from build123d import *

# Parameters (mm, degrees)
F0_W     = 70
F0_H     = 65
F1_DEPTH = 1.5
F2_W     = 5
F2_H     = 51
F3_DEPTH = 11
F4_W     = 70
F4_H     = 65
F5_DEPTH = 1.5
F6_R     = 1.5
F7_DEPTH = 25
F8_R     = 1
F9_DEPTH = 15.2


with BuildPart() as f1:
    # F0 (on Front) → F1 (new body)
    with BuildSketch(Plane.XZ):
        with Locations((35, 32.5)):
            Rectangle(F0_W, F0_H)
    extrude(amount=-F1_DEPTH)

    # F2 (on face) → F3 (join)
    with BuildSketch(Plane(origin=(0, 1.5, 0), x_dir=(-1, 0, 0), z_dir=(0, 1, 0))):
        with Locations((-67.5, 32.5)):
            Rectangle(F2_W, F2_H)
        with Locations((-2.5, 32.5)):
            Rectangle(F2_W, F2_H)
    extrude(amount=F3_DEPTH)

    # F4 (on face) → F5 (join)
    with BuildSketch(Plane(origin=(0, 12.5, 0), x_dir=(-1, 0, 0), z_dir=(0, 1, 0))):
        with Locations((-35, 32.5)):
            Rectangle(F4_W, F4_H)
    extrude(amount=F5_DEPTH)

    # F6 (on Front) → F7 (cut)
    with BuildSketch(Plane.XZ):
        with Locations((3, 62)):
            Circle(F6_R)
        with Locations((67, 62)):
            Circle(F6_R)
        with Locations((3, 3)):
            Circle(F6_R)
        with Locations((67, 3)):
            Circle(F6_R)
    extrude(amount=-F7_DEPTH, mode=Mode.SUBTRACT)

    # F8 (on face) → F9 (join)
    with BuildSketch(Plane.XZ):
        Polygon((5.75, 60.412287), (5.75, 63.587713), (3, 65.175426), (0.25, 63.587713), (0.25, 60.412287), (3, 58.824574), align=None)
        with Locations((3, 62)):
            Circle(F8_R, mode=Mode.SUBTRACT)
        Polygon((5.75, 1.412287), (5.75, 4.587713), (3, 6.175426), (0.25, 4.587713), (0.25, 1.412287), (3, -0.175426), align=None)
        with Locations((3, 3)):
            Circle(F8_R, mode=Mode.SUBTRACT)
        Polygon((67, 58.824574), (69.75, 60.412287), (69.75, 63.587713), (67, 65.175426), (64.25, 63.587713), (64.25, 60.412287), align=None)
        with Locations((67, 62)):
            Circle(F8_R, mode=Mode.SUBTRACT)
        Polygon((67, -0.175426), (69.75, 1.412287), (69.75, 4.587713), (67, 6.175426), (64.25, 4.587713), (64.25, 1.412287), align=None)
        with Locations((67, 3)):
            Circle(F8_R, mode=Mode.SUBTRACT)
    extrude(amount=F9_DEPTH)


solid = f1.part
Source: CAD feature listing. Evaluate the final solid. Frame: model axes, mm. A direction names the side the tool comes from. Round coordinates to 2 decimals unless told otherwise and drop trailing zeros. Loops run counter-clockwise (first coordinate to the right, second up) from the corner with the lowest first, then second, coordinate; pieces in that order, holes last.
Q1. Section B-B, the plane x = 58. Return loops of the section in (y, z), plus the area to 3 significant figures.
Q2. Section C-C, the plane z = 29.5. Return loops of the section in (x, y), plus the area to 3 significant figures.
Q3. Section D-D, the plane y = 4. Return loops of the section in (x, z), plus the area to 3 significant figures.
Q4. Section A-A, the plane y = -9.5. Return loops of the section in (x, z), plus the area to 3 significant figures.
Q5. First-contact query: P1, Ø12, axis at x = 14.5, z = 15.5, coming from the -Y side; P2, Ø3.5, axis at y = -11.5, z = 61.5, coming from the +X side; P3, Ø1, axis at y = -11.5, z = 61, coming from the -X side; P4, Ø4, axis at x = 3, z = 62, coming from the +Y side. Flat tips, straight axial feed; report the tip coordinate or a pass-through.
Q6. Access query for faces 5 (the face through (4.394, -7.494, 5.37)), 6 (the face through (4.36, -7.49, 0.61)), 7 (the face through (2.805, 13.24, 63.487)). Directions: +Z, -Z, +X, -X, +Y, -Y. A direction counts if a zero-diameter tool reaches every point of the face in a straight line with its end or side. Return the directions, or none.
Q7. Ray query, line 1 (Z direction, x = 3, y = -3); line 2 (Z direction, x = 3, y = 0.45); line 3 (Y direction, x = 32, z = 44). Return the intervals inside material, ascending.
Q8. Mould query, pull axis X, two halves, no side actions, for faces 1 (the face through (1.606, -7.494, 0.63)), 2 (the face through (68.394, -7.494, 64.37)), 3 (the face through (65, 7, 32)), 4 (the face through (3, 7, 58)). Classes: pulls with the +X half, pulls with the -X half, needs draft (parallel to the pull), parting line crosses it, or undercut.
Solutions:
1. outline: (0, 0) - (1.5, 0) - (1.5, 65) - (0, 65) - close; (12.5, 0) - (14, 0) - (14, 65) - (12.5, 65) - close
1. area: 195 mm2
2. outline: (0, 0) - (70, 0) - (70, 14) - (0, 14) - close; hole (5, 1.5) - (65, 1.5) - (65, 12.5) - (5, 12.5) - close
2. area: 320 mm2
3. outline: (0, 7) - (5, 7) - (5, 58) - (0, 58) - close; (65, 7) - (70, 7) - (70, 58) - (65, 58) - close
3. area: 510 mm2
4. outline: (0.25, 1.41) - (3, -0.18) - (5.75, 1.41) - (5.75, 4.59) - (3, 6.18) - (0.25, 4.59) - close; (0.25, 60.41) - (3, 58.82) - (5.75, 60.41) - (5.75, 63.59) - (3, 65.18) - (0.25, 63.59) - close; (64.25, 1.41) - (67, -0.18) - (69.75, 1.41) - (69.75, 4.59) - (67, 6.18) - (64.25, 4.59) - close; (64.25, 60.41) - (67, 58.82) - (69.75, 60.41) - (69.75, 63.59) - (67, 65.18) - (64.25, 63.59) - close; hole circle Ø2 at (3, 3); hole circle Ø2 at (3, 62); hole circle Ø2 at (67, 3); hole circle Ø2 at (67, 62)
4. area: 92.2 mm2
5. P1: stops at y = 0
5. P2: stops at x = 69.75
5. P3: stops at x = 0.25
5. P4: stops at y = 14
6. face 5: -Y
6. face 6: -Z, -Y
6. face 7: +Y
7. line 1: z = -0.18 to 2, 4 to 6.18, 58.82 to 61, 63 to 65.18
7. line 2: z = 0 to 1.5, 4.5 to 60.5, 63.5 to 65
7. line 3: y = 0 to 1.5, 12.5 to 14
8. face 1: pulls with the -X half
8. face 2: pulls with the +X half
8. face 3: undercut
8. face 4: needs draft
